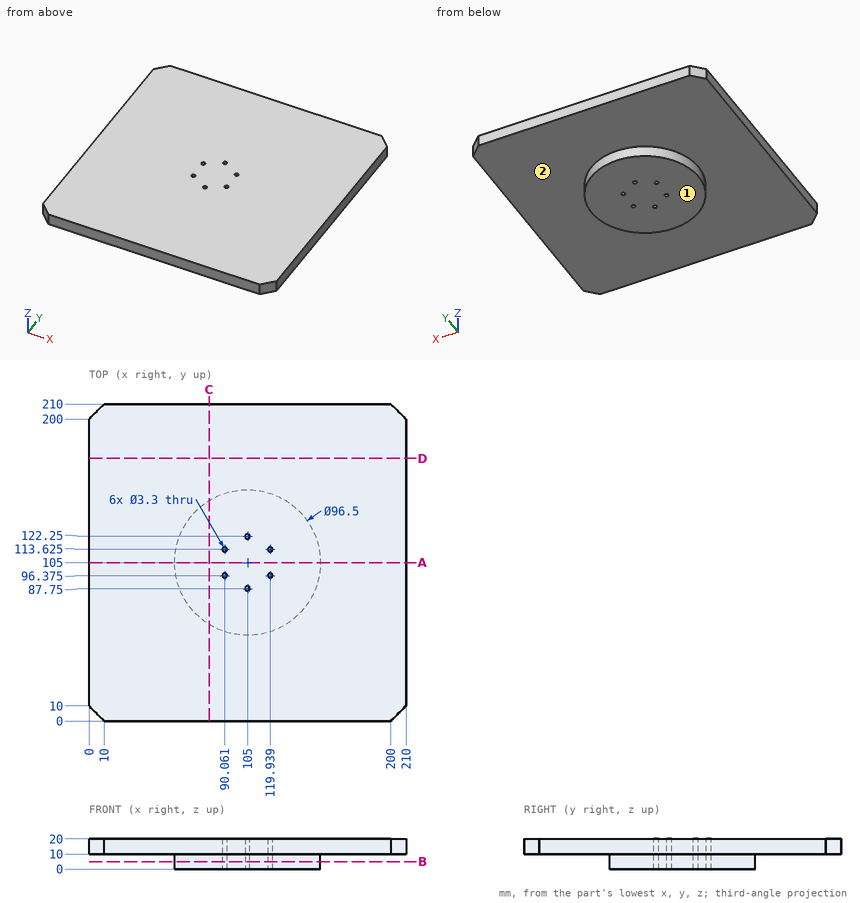
Geometry check sheet. Reference: drawing and pictorial views, mm from the part's lowest x, y, z. A direction names the side the tool comes from. Round coordinates to 2 decimals unless told otherwise and drop trailing zeros. Order: outer loops, then holes, each group sorted by start corner. A loop starts at its lowest first (then second) coordinate and runs counter-clockwise, first axis right, second up. Notation, with made-up numbers: M -27.75,6 L 8.25,6 A21 cw 8.25,33 Z; hole C 74,-4 d5. An arc over 180 degrees is marked long. Answer in a Markdown table with one row per item.
(1) Sectioned sample at C-C, the plane x = 79.5. Record the cut outline in (y, z).
Responses:
| item | result |
|---|---|
| outline | M 0,10 L 64.04,10 L 64.04,0 L 145.96,0 L 145.96,10 L 210,10 L 210,20 L 0,20 Z |
(2) Sectioned sample at B-B, the plane z = 5. Record the cut outline in (x, y) (3 decimals), and give its area (3 significant figures).
Responses:
| item | result |
|---|---|
| outline | C 105,105 d96.5; hole C 90.061,96.375 d3.3; hole C 90.061,113.625 d3.3; hole C 105,87.75 d3.3; hole C 105,122.25 d3.3; hole C 119.939,96.375 d3.3; hole C 119.939,113.625 d3.3 |
| area | 7,260 mm² |
(3) Tool access check on the marked faces 1 and 2. Record the directions out of +Z, -Z, +X, -X, +Y, -Y that give a thin tool (end or side, any length) a straight path to the whole face; none if there is none.
Responses:
| item | result |
|---|---|
| face 1 | -Z, +X, -X, +Y, -Y |
| face 2 | -Z |
(4) Go/stop test with a flat-tipped pin: P1, Ø12, axis at x = 108.5, y = 36, coming from the -Z side. Record where the tip stops, or that it passes through.
Responses:
| item | result |
|---|---|
| P1 | stops at z = 10 |
(5) Sectioned sample at A-A, the plane y = 105. Record the cut outline in (x, z).
Responses:
| item | result |
|---|---|
| outline | M 0,10 L 56.75,10 L 56.75,0 L 153.25,0 L 153.25,10 L 210,10 L 210,20 L 0,20 Z |
(6) Scan lines: probe 1 along Y at (x, z) = (105, 7.25); probe 2 along X at (y, z) = (122.25, 12); probe 3 along Z at (x, y) = (158, 25.5). Record each from-to range of solid material in increasing order. Write a range as from..to.
Responses:
| item | result |
|---|---|
| probe 1 | y = 56.75..86.1, 89.4..120.6, 123.9..153.25 |
| probe 2 | x = 0..103.35, 106.65..210 |
| probe 3 | z = 10..20 |
(7) Sectioned sample at D-D, the plane y = 174. Record the cut outline in (x, z), and give its area (3 significant figures).
Responses:
| item | result |
|---|---|
| outline | M 0,10 L 210,10 L 210,20 L 0,20 Z |
| area | 2,100 mm² |
